Work out the finished part from the listing and answer in its coordinate system (mm). Face numbers are marked on the shaded views. A direction names the side the tool comes from. Give positions to 0.01 mm unless a question says otherwise; leave off trailing zeros. Order: outer loops, then holes, each group sorted by start corner. A loop starts at its lowest first (then second) coordinate and runs counter-clockwise, first axis right, second up. Notation, with made-up numbers: M -7.5,34.25 L -0.5,34.25 A23 cw -0.5,70.25 Z; hole C 83,46 d4. An arc over 180 degrees is marked long. One line per item, written item: value.
from build123d import *

# Parameters (mm, degrees)
F2_DEPTH = 10


# Not quite as in the source:
# - a feature names something its author has since deleted; it is built from what else it names


with BuildPart() as f2:
    # F1 (on Top) → F2 (new body)
    with BuildSketch(Plane.XY):
        with BuildLine():
            ThreePointArc((-20.7961524227, -0.7545254038), (-18.6080572337, 1.3728200267), (-16.1, 3.1115))
            Line((-16.1, 3.1115), (-11.6, -4.6827286341))
            ThreePointArc((-11.6, -4.6827286341), (-14.3597696428, -5.9854299259), (-17.2961524227, -6.8167032303))
            Line((-17.2961524227, -6.8167032303), (-18.0461524227, -5.5176651246))
            Line((-18.0461524227, -5.5176651246), (-18.7389727457, -5.9176651246))
            Line((-18.7389727457, -5.9176651246), (-17.7077768116, -7.703748875))
            ThreePointArc((-17.7077768116, -7.703748875), (-13.9735101965, -6.69466899), (-10.5154733964, -4.9611838136))
            Line((-10.5154733964, -4.9611838136), (-10, -4.9611838136))
            Line((-10, -4.9611838136), (-10, -3.3615))
            Line((-10, -3.3615), (-8.722, -3.3615))
            Line((-8.722, -3.3615), (-8.222, -4.1115))
            Line((-8.222, -4.1115), (-7.822, -4.1115))
            Line((-7.822, -4.1115), (-6.222, -2.5115))
            Line((-6.222, -2.5115), (-6.222, -1.5115))
            Line((-6.222, -1.5115), (-10, -1.5115))
            ThreePointArc((-10, -1.5115), (-10.319496099, -1.5437237906), (-10.6261229788, -1.6390971966))
            ThreePointArc((-10.6261229788, -1.6390971966), (-13.1042708913, 0), (-10.6261229788, 1.6390971966))
            ThreePointArc((-10.6261229788, 1.6390971966), (-10.319496099, 1.5437237906), (-10, 1.5115))
            Line((-10, 1.5115), (-6.222, 1.5115))
            Line((-6.222, 1.5115), (-6.222, 2.5115))
            Line((-6.222, 2.5115), (-7.822, 4.1115))
            Line((-7.822, 4.1115), (-8.222, 4.1115))
            Line((-8.222, 4.1115), (-8.722, 3.3615))
            Line((-8.722, 3.3615), (-10, 3.3615))
            Line((-10, 3.3615), (-10, 4.1899551795))
            Line((-10, 4.1899551795), (-10, 6.131235349))
            ThreePointArc((-10, 6.131235349), (-12.9768183038, 5.3917266036), (-15.7988859575, 4.1899551795))
            ThreePointArc((-15.7988859575, 4.1899551795), (-19.0291465574, 2.0619500516), (-21.7701686798, -0.6674797591))
            Line((-21.7701686798, -0.6674797591), (-20.7389727457, -2.4535635095))
            Line((-20.7389727457, -2.4535635095), (-20.0461524227, -2.0535635095))
            Line((-20.0461524227, -2.0535635095), (-20.7961524227, -0.7545254038))
        make_face()
    extrude(amount=F2_DEPTH)


solid = f2.part
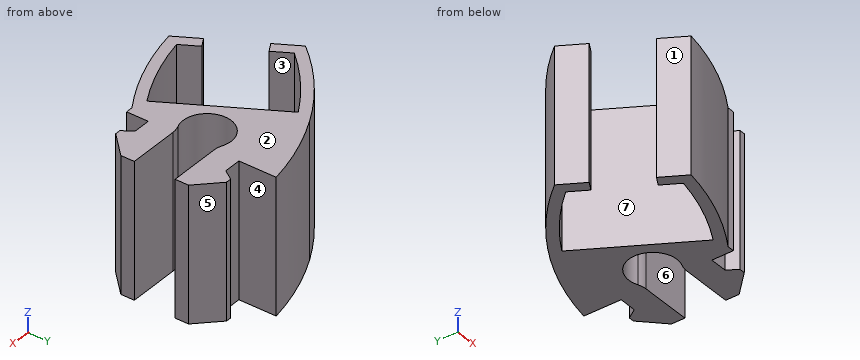
(1) Which of the six approach directions +Z, -Z, +X, -X, +Y, -Y give full straight-line access (tool end or side, diameter ignored) to the marked faces 4, 5, 6 and 7?
Findings:
face 4: +Z, -Z, +Y
face 5: +Z, -Z, +X, +Y
face 6: +Z, -Z, +X
face 7: +Z, -Z
(2) Section B-B, the plane y = -1 is taken. Give the vertices of the cut face in (x, z), then the cut area to 3 significant figures.
Findings:
outline: M -21.58,0 L -20.65,0 L -20.65,10 L -21.58,10 Z; M -13.73,0 L -12.8,0 L -12.8,10 L -13.73,10 Z
area: 18.5 mm^2
(3) Section C-C, the plane x = -8.5 is taken. Give the vertices of the cut face in (y, z).
Findings:
outline: M -3.69,0 L -1.51,0 L -1.51,10 L -3.69,10 Z; M 1.51,0 L 3.69,0 L 3.69,10 L 1.51,10 Z
(4) Find the intervals of material crossed by probe 1 along Y at (x, z) = (-9, 7.25); probe 2 along X at (y, z) = (-1.25, 2.5); probe 3 along Y at (x, z) = (-11, 5.5), in increasing order. Write a range as from..to.
Findings:
probe 1: y = -3.36..-1.51, 1.51..3.36
probe 2: x = -21.43..-20.51, -13.58..-12.59
probe 3: y = -5.26..-1.75, 1.75..5.94
(5) Determine the mould class of the marked faces 1, 2 and 3 for opening direction Y: pulls with the +Y half, pulls with the -Y half, needs draft (parallel to the pull), parting line crosses it, or undercut.
Findings:
face 1: pulls with the -Y half
face 2: needs draft
face 3: undercut
(6) Given P1, Ø1.9, axis at x = -9, z = 3, coming from the -Y side; P2, Ø1.9, axis at x = -7.5, z = 4, coming from the +Y side, each flat-ended and moving along its own axis, determine where each tip first touches the part or whether it passes through.
Findings:
P1: stops at y = -4.11
P2: stops at y = 4.11
